Build history of the part. All positions in model axes, mm. Face numbers are marked on the shaded views. A direction names the side the tool comes from. Coordinates: 2 decimals unless noted, no trailing zeros. Order: outer loops, then holes, each group sorted by start corner. A loop starts at its lowest first (then second) coordinate and runs counter-clockwise, first axis right, second up. Notation, with made-up numbers: M 2,-9 L 46,-9 A14 cw 46,7 Z; hole C -36.5,-23 d11. An arc over 180 degrees is marked long. Write item = value, one per line. Start each with the question number.
Q1. Band-saw the part on A-A on y = 9.25. Write the cut outline in (x, z), plus the area to 3 significant figures.
Q2. Band-saw the part on D-D on y = 17.25. Write the cut outline in (x, z).
Q3. Pull direction Y, two halves, no side cores. Call the marked faces 4, 5 and 6: released by +Y, released by -Y, zero draft, split by the parting line, or undercut.
Q4. Pin check, flat tips, straight feed: P1, Ø1, axis at x = 52.5, y = 16, coming from the -Z side; P2, Ø2, axis at x = 35, y = 3.5, coming from the +Z side; P3, Ø6, axis at x = 27.5, y = 10.5, coming from the -Z side. Stop position of each tip, or through.
Q5. Drill centre lines: probe 1 along X at (y, z) = (9.25, 38.5); probe 2 along X at (y, z) = (17.5, 21); probe 3 along X at (y, z) = (8, 27.5). Where is each one in solid material? Low to high.
Q6. Band-saw the part on C-C on z = 34. Write the cut outline in (x, y).
Q7. Band-saw the part on B-B on x = 23. Write the cut outline in (y, z).
Q8. 3-axis set-ups, long thin cutter, end or side, ignore diameter. For the marked faces 1, 2 and 3: which of +Z, -Z, +X, -X, +Y, -Y reach the whole face in a straight line?
```python
from build123d import *

# Parameters (mm, degrees)
BOSS_EXTRUDE1_DEPTH     = 18.5
SKETCH2_W               = 18.5
SKETCH2_H               = 13.212440144
BOSS_EXTRUDE2_DEPTH     = 9.25
SKETCH4_R               = 5.25
CUT_EXTRUDE1_DEPTH      = 65.978958769
CUT_EXTRUDE1_DEPTH_BACK = 36.75
BOSS_EXTRUDE3_DEPTH     = 9.25
CUT_EXTRUDE3_START      = 5
SKETCH5_R               = 6.5
CUT_EXTRUDE3_DEPTH      = 11.5
SKETCH7_W               = 10
SKETCH7_H               = 4
BOSS_EXTRUDE4_DEPTH     = 10
SKETCH8_W               = 10
SKETCH8_H               = 4
BOSS_EXTRUDE5_DEPTH     = 10
SKETCH9_R               = 1.25
CUT_EXTRUDE4_DEPTH      = 1
CUT_EXTRUDE4_DEPTH_BACK = 19.5
CUT_EXTRUDE5_REACH      = 20.5


with BuildPart() as part:
    # Sketch1 → Boss-Extrude1 (new body)
    with BuildSketch(Plane(origin=(0, 0, 0), x_dir=(1, 0, 0), z_dir=(0, 1, 0))):
        Polygon((0, 0), (0, 5.75), (3.6, 5.75), (77.618084718, -94.978958769), (69.792845102, -94.978958769), align=None)
    extrude(amount=BOSS_EXTRUDE1_DEPTH)

    # Sketch2 → Boss-Extrude2 (add, symmetric)
    with BuildSketch(Plane(origin=(0, 9.25, 0), x_dir=(1, 0, 0), z_dir=(0, 1, 0))):
        with Locations((25.134167429, -29.209707688)):
            Rectangle(SKETCH2_W, SKETCH2_H)
    extrude(amount=BOSS_EXTRUDE2_DEPTH, both=True)

    # Sketch4 → Cut-Extrude1 (cut, two sides)
    with BuildSketch(Plane.XY.offset(30)) as cut_extrude1_sk:
        with Locations((25.134167429, 9.25)):
            Circle(SKETCH4_R)
    extrude(amount=CUT_EXTRUDE1_DEPTH, mode=Mode.SUBTRACT)
    extrude(cut_extrude1_sk.sketch, amount=-CUT_EXTRUDE1_DEPTH_BACK, mode=Mode.SUBTRACT)

    # Sketch6 → Boss-Extrude3 (add, symmetric)
    with BuildSketch(Plane(origin=(0, 9.25, 0), x_dir=(1, 0, 0), z_dir=(0, 1, 0))):
        with BuildLine():
            Line((34.384167429, -22.603487616), (34.143652987, -35.81592776))
            Line((34.143652987, -35.81592776), (47.347337909, -53.784420719))
            ThreePointArc((47.347337909, -53.784420719), (47.065802481, -35.616343599), (34.384167429, -22.603487616))
        make_face()
    extrude(amount=BOSS_EXTRUDE3_DEPTH, both=True)

    # Sketch5 → Cut-Extrude3 (cut)
    with BuildSketch(Plane.XY.offset(30).offset(CUT_EXTRUDE3_START)):
        with Locations((25.150542623, 9.25)):
            Circle(SKETCH5_R)
    extrude(amount=CUT_EXTRUDE3_DEPTH, mode=Mode.SUBTRACT)

    # Sketch7 → Boss-Extrude4 (add)
    with BuildSketch(Plane(origin=(0, 0, 0), x_dir=(0.592144678, 0, 0.80583167), z_dir=(-0.80583167, 0, 0.592144678))):
        with Locations((18.049887406, 2)):
            Rectangle(SKETCH7_W, SKETCH7_H)
        with Locations((18.049887406, 16.5)):
            Rectangle(SKETCH7_W, SKETCH7_H)
    extrude(amount=BOSS_EXTRUDE4_DEPTH)

    # Sketch8 → Boss-Extrude5 (add)
    with BuildSketch(Plane(origin=(0, 0, 0), x_dir=(0.592144678, 0, 0.80583167), z_dir=(-0.80583167, 0, 0.592144678))):
        with Locations((86.155216017, 2)):
            Rectangle(SKETCH8_W, SKETCH8_H)
        with Locations((86.155216017, 16.5)):
            Rectangle(SKETCH8_W, SKETCH8_H)
    extrude(amount=BOSS_EXTRUDE5_DEPTH)

    # Sketch9 → Cut-Extrude4 (cut, two sides)
    with BuildSketch(Plane(origin=(0, 18.5, 0), x_dir=(1, 0, 0), z_dir=(0, 1, 0))) as cut_extrude4_sk:
        with Locations((6.65898641, -17.505894303)):
            Circle(SKETCH9_R)
        with Locations((46.987194274, -72.387325004)):
            Circle(SKETCH9_R)
    extrude(amount=CUT_EXTRUDE4_DEPTH, mode=Mode.SUBTRACT)
    extrude(cut_extrude4_sk.sketch, amount=-CUT_EXTRUDE4_DEPTH_BACK, mode=Mode.SUBTRACT)

    # Sketch10 → Cut-Extrude5 (cut, up to next)
    with BuildSketch(Plane(origin=(0, 18.5, 0), x_dir=(1, 0, 0), z_dir=(0, 1, 0)), mode=Mode.PRIVATE) as cut_extrude5_sk1:
        Polygon((69.792845102, -84.329828334), (69.792845102, -94.978958769), (77.618084718, -94.978958769), align=None)
    cut_extrude5_tool1 = extrude(cut_extrude5_sk1.sketch, amount=-CUT_EXTRUDE5_REACH, mode=Mode.PRIVATE) & part.part
    add(cut_extrude5_tool1.solids().sort_by_distance((72.401258, 18.5, 91.429249))[0], mode=Mode.SUBTRACT)


solid = part.part
```
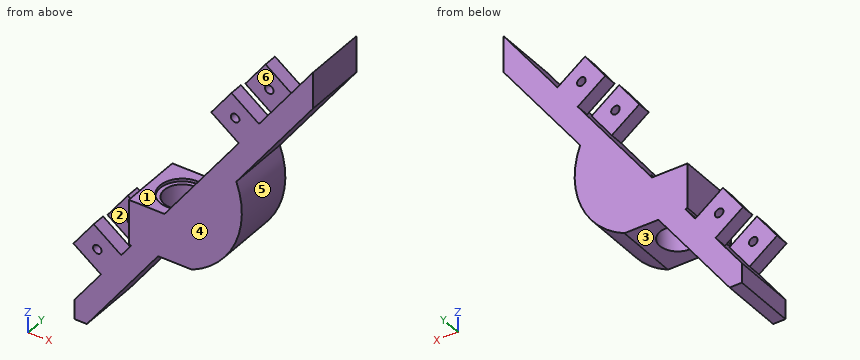
Recorded:
q1.outline = M 0,-5.75 L 3.6,-5.75 L 19.88,16.41 L 19.88,35 L 18.65,35 L 18.65,35.82 L 15.88,35.82 L 15.88,22.6 L 16.61,22.6 L 0,0 Z; M 30.38,22.6 L 34.38,22.6 A24.59 ccw 47.35,53.78 L 69.79,84.33 L 69.79,94.98 L 31.65,43.07 L 31.65,35 L 30.38,35 Z
q1.area = 945 mm2
q2.outline = M -0.33,16.44 L 7.73,10.52 L 0,0 L 0,-5.75 L 3.6,-5.75 L 24.43,22.6 L 34.38,22.6 A24.59 ccw 47.35,53.78 L 69.79,84.33 L 69.79,94.98 L 53.98,73.46 L 45.92,79.38 L 40,71.32 L 48.06,65.4 L 26.32,35.82 L 15.88,35.82 L 15.88,22.6 L 16.61,22.6 L 13.65,18.57 L 5.59,24.5 Z; hole C 6.66,17.51 d2.5; hole C 46.99,72.39 d2.5
q3.face_4 = released by -Y
q3.face_5 = zero draft
q3.face_6 = undercut
q4.P1 = 60.12
q4.P2 = 48.99
q4.P3 = 22.6
q5.probe_1 = 31.65 to 48.06
q5.probe_2 = 3.02 to 10.35, 15.43 to 23.26
q5.probe_3 = 15.88 to 20.04, 30.23 to 41.58
q6.outline = M 15.88,0 L 46.32,0 L 46.32,18.5 L 15.88,18.5 Z; hole C 25.13,9.25 d10.5
q7.outline = M 0,20.65 L 4.45,20.65 L 4.45,35 L 3.12,35 L 3.12,35.82 L 0,35.82 Z; M 14.05,20.65 L 18.5,20.65 L 18.5,35.82 L 15.38,35.82 L 15.38,35 L 14.05,35 Z
q8.face_1 = +Z, -X, +Y, -Y
q8.face_2 = +Z, -X
q8.face_3 = -Z, +X, +Y, -Y
